Could you check a few things on this model? Use its own coordinates, in mm. A direction names the side the tool comes from. Round coordinates to 2 decimals unless told otherwise and drop trailing zeros. Loops run counter-clockwise (first coordinate to the right, second up) from the corner with the lowest first, then second, coordinate; pieces in that order, holes last. Notation, with made-up numbers: (31, 61.5) -> (40, 61.5) arc R19 ccw to (40, 72.5) -> close; hole circle Ø10 at (53, -33.5). An arc over 180 degrees is marked (long way). Put each result on its own line as item: value. Start each with the question number.
1. I need wall thicknesses on line 1 (X direction, y = 75, z = 0); line 2 (Y direction, x = 0, z = -0.25); line 3 (X direction, y = 98.5, z = -5.25). Which ranges of each line are inside material? Lowest first, please. Write a range as [from, to].
2. I'm going to push flat-ended pins straight in: P1, Ø0.8, axis at x = -0.5, z = -8, coming from the -Y side; P2, Ø8.5, axis at x = 0, y = 75, coming from the +Z side; P3, Ø1, axis at y = 48.5, z = -4, coming from the -X side. Where does each tip first touch, or does it pass through?
3. Imagine slicing it at B-B, the plane z = 0. Please give me the cut outline in (x, y).
4. If we mould it in two halves opening along Y, with no side actions, what happens to faces 1 (the cylindrical face through (3.577, 76.126, 0.105)), 2 (the flat face through (0, 0, 0)), 3 (the flat face through (0, 105, 0))? For each: pulls with the +Y half, pulls with the -Y half, needs draft (parallel to the pull), parting line crosses it, or undercut.
5. Which directions (+Z, -Z, +X, -X, +Y, -Y) give clear straight access to the entire face, cutting with the end or side of a thin tool? Please do faces 4 (the flat face through (-1.5, 100, 0)), 5 (the flat face through (0, 95, 9)).
6. Imagine slicing it at C-C, the plane y = 96. Please give me the cut outline in (x, z).
7. Imagine slicing it at A-A, the plane x = 0. Please give me the cut outline in (y, z), and give its area (3 significant figures).
8. Imagine slicing it at D-D, the plane z = -4.5. Please give me the cut outline in (x, y), and give its area (3 significant figures).
```python
from build123d import *

# Parameters (mm, degrees)
SKETCH1_R               = 7.5
BOSS_EXTRUDE1_DEPTH     = 105
SKETCH2_R               = 3.75
CUT_EXTRUDE1_DEPTH      = 8.5
CUT_EXTRUDE1_DEPTH_BACK = 8.5
SKETCH3_R               = 2.5
CUT_EXTRUDE2_DEPTH      = 10
CUT_EXTRUDE2_DEPTH_BACK = 10
SKETCH4_W               = 3
SKETCH4_H               = 18
BOSS_EXTRUDE2_DEPTH     = 20


with BuildPart() as part:
    # Sketch1 → Boss-Extrude1 (new body)
    with BuildSketch(Plane(origin=(0, 0, 0), x_dir=(1, 0, 0), z_dir=(0, 1, 0))):
        Circle(SKETCH1_R)
    extrude(amount=BOSS_EXTRUDE1_DEPTH)

    # Sketch2 → Cut-Extrude1 (cut, two sides)
    with BuildSketch(Plane.XY) as cut_extrude1_sk:
        with Locations((0, 75)):
            Circle(SKETCH2_R)
    extrude(amount=CUT_EXTRUDE1_DEPTH, mode=Mode.SUBTRACT)
    extrude(cut_extrude1_sk.sketch, amount=-CUT_EXTRUDE1_DEPTH_BACK, mode=Mode.SUBTRACT)

    # Sketch3 → Cut-Extrude2 (cut, two sides)
    with BuildSketch(Plane.XY) as cut_extrude2_sk:
        with Locations((0, 100)):
            Circle(SKETCH3_R)
    extrude(amount=CUT_EXTRUDE2_DEPTH, mode=Mode.SUBTRACT)
    extrude(cut_extrude2_sk.sketch, amount=-CUT_EXTRUDE2_DEPTH_BACK, mode=Mode.SUBTRACT)

    # Sketch4 → Boss-Extrude2 (add)
    with BuildSketch(Plane(origin=(0, 105, 0), x_dir=(1, 0, 0), z_dir=(0, 1, 0))):
        Rectangle(SKETCH4_W, SKETCH4_H)
    extrude(amount=-BOSS_EXTRUDE2_DEPTH)


solid = part.part
```
Entries:
1. line 1: [-7.5, -3.75], [3.75, 7.5]
1. line 2: [0, 71.25], [78.75, 105]
1. line 3: [-5.36, -2], [-1.5, 1.5], [2, 5.36]
2. P1: y = 85
2. P2: z = 7.5
2. P3: x = -6.63
3. outline: (-7.5, 0) -> (7.5, 0) -> (7.5, 105) -> (-7.5, 105) -> close; hole circle Ø7.5 at (0, 75); hole (-1.5, 98) -> (-1.5, 102) arc R2.5 ccw to start; hole (1.5, 98) arc R2.5 ccw to (1.5, 102) -> close
4. face 1: undercut
4. face 2: pulls with the -Y half
4. face 3: pulls with the +Y half
5. face 4: none
5. face 5: +Z, +X, -X, +Y, -Y
6. outline: (-1.5, -9) -> (1.5, -9) -> (1.5, -7.35) arc R7.5 ccw to (1.5, 7.35) -> (1.5, 9) -> (-1.5, 9) -> (-1.5, 7.35) arc R7.5 ccw to (-1.5, -7.35) -> close
7. outline: (0, -7.5) -> (71.25, -7.5) -> (71.25, 7.5) -> (0, 7.5) -> close; (78.75, -7.5) -> (85, -7.5) -> (85, -9) -> (105, -9) -> (105, 9) -> (85, 9) -> (85, 7.5) -> (78.75, 7.5) -> close
7. area: 1,520 mm^2
8. outline: (-6, 0) -> (6, 0) -> (6, 105) -> (-6, 105) -> close; hole circle Ø7.5 at (0, 75); hole (-1.5, 98) -> (-1.5, 102) arc R2.5 ccw to start; hole (1.5, 98) arc R2.5 ccw to (1.5, 102) -> close
8. area: 1,210 mm^2
